The drawing under review shows one solid part. Ordinate dimensions are in mm from its lowest x, y, z. Coordinates: 2 decimals unless noted, no trailing zeros. Loops run counter-clockwise (first coordinate to the right, second up) from the corner with the lowest first, then second, coordinate; pieces in that order, holes last. Notation, with made-up numbers: M 9.25,53 L 52.25,53 A28 cw 52.25,81 Z; hole C 79.5,35.25 d8. An arc over 180 degrees is marked long. Put each result on its own line as item: value.
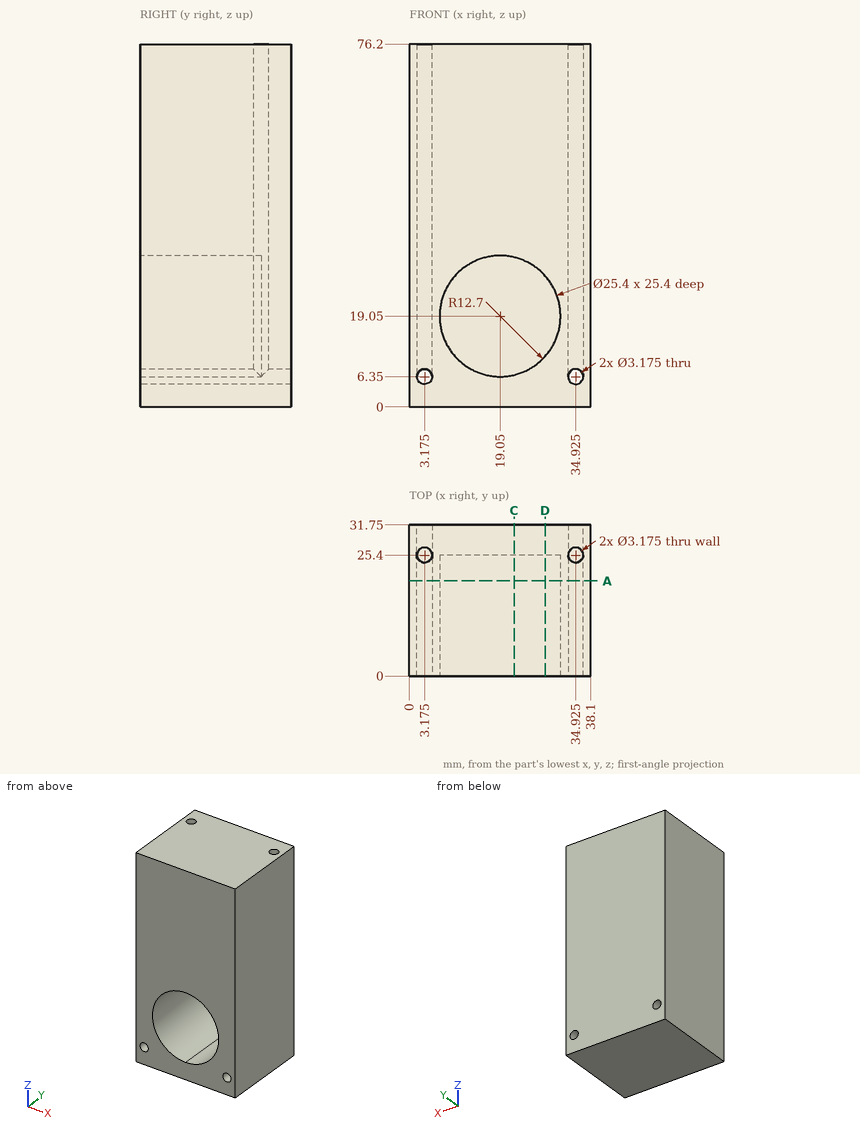
(1) Add section D-D (x = 28.5). Write out the cut boundary in (y, z), plus the area to 3 significant figures.
Determined:
outline: M 0,0 L 31.75,0 L 31.75,76.2 L 0,76.2 L 0,27.53 L 25.4,27.53 L 25.4,10.57 L 0,10.57 Z
area: 1,990 mm^2
(2) Add section A-A (y = 20). State how many separate pieces and enclosed holes the cut face has, plus the area to 3 significant figures.
Determined:
separate pieces: 1
enclosed holes: 3
area: 2,380 mm^2
(3) Wall thickness on line 1 along X through (y, z) = (25.4, 51); line 2 along Z through (x, y) = (19, 8); line 3 along Z through (x, y) = (29.5, 14.5): over which ranges is each line inside the solid? List them lowest first. Write a range as [from, to].
Determined:
line 1: x = [0, 1.59], [4.76, 33.34], [36.51, 38.1]
line 2: z = [0, 6.35], [31.75, 76.2]
line 3: z = [0, 11.83], [26.27, 76.2]
(4) Add section C-C (x = 22). Write out the cut boundary in (y, z).
Determined:
outline: M 0,0 L 31.75,0 L 31.75,76.2 L 0,76.2 L 0,31.4 L 25.4,31.4 L 25.4,6.7 L 0,6.7 Z
